Build history of the part. All positions in model axes, mm. Face numbers are marked on the shaded views. A direction names the side the tool comes from. Round coordinates to 2 decimals unless told otherwise and drop trailing zeros. Write each loop counter-clockwise with the first axis right and the second up, starting at its lowest first coordinate (ties: lowest second). Pieces come first, ordered by that corner, then holes. Notation, with made-up numbers: M 74,63 L 129,63 A25 cw 129,89 Z; hole C -22.75,79 d3. An arc over 180 degrees is marked long. Use a Markdown table: item, result.
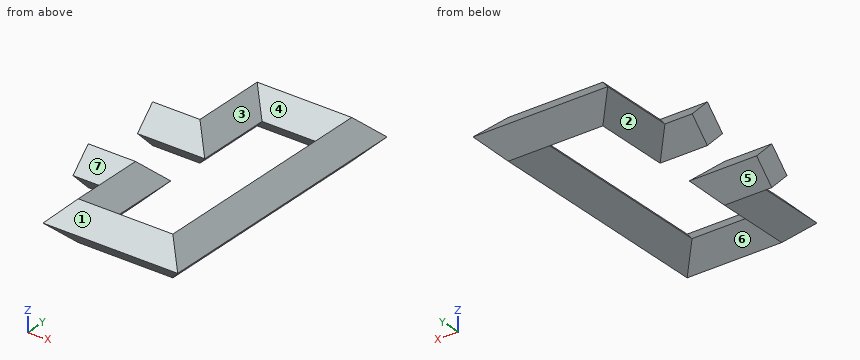
from build123d import *


with BuildPart() as part:
    # 스윕1: sweep along a path in 스케치2
    with BuildLine(Plane.XY) as sweep_1_path:
        Line((0, 0), (50, 0))
        Line((50, 0), (50, 80))
        Line((50, 80), (150, 80))
        Line((150, 80), (150, -170))
        Line((150, -170), (50, -170))
        Line((50, -170), (50, -90))
        Line((50, -90), (0, -90))
    # 스케치3 → 스윕1 (sweep)
    with BuildSketch(Plane(origin=(0, 0, 0), x_dir=(0, 0, -1), z_dir=(1, 0, 0))):
        Polygon((21.213203436, 0), (0, -21.213203436), (-21.213203436, 0), (0, 21.213203436), align=None)
    sweep(path=sweep_1_path.line, transition=Transition.RIGHT)


solid = part.part
Q1. Drill centre lines: L1, parallel to X at y = 15.5, z = 4; L2, parallel to Y at x = 126, z = 15; L3, parallel to Y at x = 99, z = 5. Where is each one in solid material? Low to high.
Response values:
| item | result |
|---|---|
| L1 | x = 0 to 67.21, 132.79 to 167.21 |
| L2 | y = -176.21 to -163.79, 73.79 to 86.21 |
| L3 | y = -186.21 to -153.79, 63.79 to 96.21 |
Q2. Cut at B-B on x = 117.5. Give the cut face in (y, z).
Response values:
| item | result |
|---|---|
| outline | M -191.21,0 L -170,-21.21 L -148.79,0 L -170,21.21 Z; M 58.79,0 L 80,-21.21 L 101.21,0 L 80,21.21 Z |
Q3. Cut at A-A on y = -130.5. Give the cut face in (x, z), and give its area (3 significant figures).
Response values:
| item | result |
|---|---|
| outline | M 28.79,0 L 50,-21.21 L 71.21,0 L 50,21.21 Z; M 128.79,0 L 150,-21.21 L 171.21,0 L 150,21.21 Z |
| area | 1,800 mm2 |
Q4. Two-plate mould, pull along X, no slides. Class the marked faces 1, 2 and 3: +X half, -X half, draft (parallel to the pull), parting line (faces both ways), or undercut.
Response values:
| item | result |
|---|---|
| face 1 | draft |
| face 2 | -X half |
| face 3 | undercut |
Q5. Drop flat-ended pins along their axis: P1, Ø1.5, axis at y = -30, z = 1, coming from the +X side; P2, Ø8, axis at y = -6, z = 5, coming from the -X side; P3, Ø5, axis at x = 144.5, y = -30.5, coming from the -Z side; P4, Ø10, axis at x = 59.5, y = -111, coming from the -Z side. Give the stop position or say it passes through.
Response values:
| item | result |
|---|---|
| P1 | stops at x = 170.96 |
| P2 | stops at x = 0 |
| P3 | stops at z = -18.21 |
| P4 | stops at z = -16.71 |
Q6. Cut at D-D on z = -4. Give the cut face in (x, y).
Response values:
| item | result |
|---|---|
| outline | M 0,-107.21 L 32.79,-107.21 L 32.79,-187.21 L 167.21,-187.21 L 167.21,97.21 L 32.79,97.21 L 32.79,17.21 L 0,17.21 L 0,-17.21 L 67.21,-17.21 L 67.21,62.79 L 132.79,62.79 L 132.79,-152.79 L 67.21,-152.79 L 67.21,-72.79 L 0,-72.79 Z |
Q7. Cut at C-C on y = -84. Give the cut face in (x, z).
Response values:
| item | result |
|---|---|
| outline | M 0,-15.21 L 56,-15.21 L 71.21,0 L 56,15.21 L 0,15.21 Z; M 128.79,0 L 150,-21.21 L 171.21,0 L 150,21.21 Z |
Q8. Which spindle directions (+Z, -Z, +X, -X, +Y, -Y) get a long thin tool onto all of the face, cutting with end or side? Do the marked faces 4, 5, 6 and 7. Say none if no direction does.
Response values:
| item | result |
|---|---|
| face 4 | +Z |
| face 5 | -Z, -X |
| face 6 | -Z |
| face 7 | +Z, -X, -Y |
